Read the model definition and answer for the solid it produces. Units are mm, in the model's axes. Face numbers are marked on the shaded views. A direction names the side the tool comes from. Give positions to 0.01 mm unless a question says otherwise; leave off trailing zeros. Order: outer loops, then holes, each group sorted by start corner. A loop starts at its lowest first (then second) coordinate and runs counter-clockwise, first axis right, second up. Notation, with made-up numbers: (7, 56) -> (43, 56) arc R33 ccw to (43, 85) -> close; hole circle Ø2 at (65, 20.25). An arc over 180 degrees is marked (long way). Answer as CSV lines item,"result". Start each with the question number.
1) Find section A-A (x = 0). Determine the outline of the cut face in (y, z).
2) Find section D-D (y = -6.5). Determine the outline of the cut face in (x, z), and give its area (3 significant figures).
3) For the marked faces 4, 5 and 6, determine the directions among +Z, -Z, +X, -X, +Y, -Y from which every point of the face is accessible in a straight line to the end or side of a thin tool.
4) Find section C-C (x = -20.5). Determine the outline of the cut face in (y, z), and give its area (3 significant figures).
5) Straight lines are drawn through the part: L1, parallel to Z at x = -23, y = -10.35; L2, parallel to Z at x = -2, y = 18; L3, parallel to Z at x = 6, y = 2.5. For each, find the intervals that lie inside material, in ascending order. Write a range as from..to.
6) Flat-ended cylindrical pins translate along their axes: pin 1 Ø10 at (x, z) = (0.5, 41.5) entering from +Y; pin 2 Ø5 at (y, z) = (-10.5, 22) entering from -X; pin 3 Ø9.5 at (x, z) = (-18.5, 20.5) entering from +Y. Find the tip coordinate at first contact, or state that the pin passes through.
7) The mould has two halves that part along Y. Classify the marked faces 1, 2 and 3: +Y half, -Y half, draft (parallel to the pull), parting line (faces both ways), or undercut.
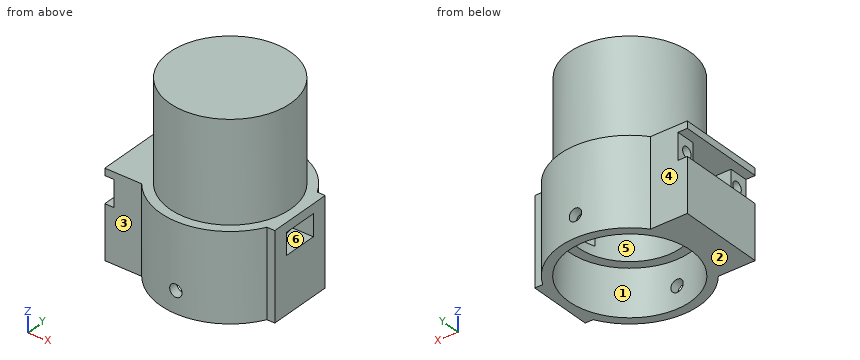
```python
from build123d import *

# Parameters (mm, degrees)
SKETCH_R        = 19.6
PAD_DEPTH       = 15
SKETCH001_R     = 16.5
PAD001_DEPTH    = 13
SKETCH002_W     = 11
SKETCH002_H     = 7
POCKET_DEPTH    = 10
SKETCH003_W     = 28
SKETCH003_H     = 8.5
POCKET001_DEPTH = 3
SKETCH004_R     = 1.75
SKETCH004_W     = 15.8
SKETCH004_H     = 8.5
POCKET002_DEPTH = 12
SKETCH006_R     = 2
HOLE_DEPTH      = 22.501
SKETCH007_R     = 2
HOLE001_DEPTH   = 22.501
SKETCH008_R     = 19.5
SKETCH008_R_2   = 16.5
PAD002_DEPTH    = 29
SKETCH009_R     = 19.5
PAD003_DEPTH    = 3


with BuildPart() as part:
    # Sketch → Pad (new body)
    with BuildSketch(Plane.XY):
        with BuildLine():
            Line((-29.5, 14), (-29.5, -14))
            Line((-29.5, -14), (-17.613915, -14))
            ThreePointArc((-17.613915, -14), (2.146366, -22.397391), (19.952193, -10.4))
            Line((19.952193, -10.4), (22.5, -10.4))
            Line((22.5, -10.4), (22.5, 10.4))
            Line((22.5, 10.4), (19.952193, 10.4))
            ThreePointArc((19.952193, 10.4), (2.146366, 22.397391), (-17.613915, 14))
            Line((-17.613915, 14), (-29.5, 14))
        make_face()
        Circle(SKETCH_R, mode=Mode.SUBTRACT)
    extrude(amount=PAD_DEPTH)

    # Sketch001 (on Face11 of Pad) → Pad001 (join)
    with BuildSketch(Plane.XY.offset(15)):
        with BuildLine():
            ThreePointArc((19.952193, 10.4), (2.146366, 22.397391), (-17.613915, 14))
            Line((-17.613915, 14), (-29.5, 14))
            Line((-29.5, 14), (-29.5, -14))
            Line((-29.5, -14), (-17.613915, -14))
            ThreePointArc((-17.613915, -14), (2.146366, -22.397391), (19.952193, -10.4))
            Line((22.5, -10.4), (19.952193, -10.4))
            Line((22.5, 10.4), (22.5, -10.4))
            Line((19.952193, 10.4), (22.5, 10.4))
        make_face()
        Circle(SKETCH001_R, mode=Mode.SUBTRACT)
    extrude(amount=PAD001_DEPTH)

    # Sketch002 (on Face10 of Pad001) → Pocket (cut)
    with BuildSketch(Plane.YZ.offset(22.5)):
        with Locations((0, 21.5)):
            Rectangle(SKETCH002_W, SKETCH002_H)
    extrude(amount=-POCKET_DEPTH, mode=Mode.SUBTRACT)

    # Sketch003 (on Face2 of Pocket) → Pocket001 (cut)
    with BuildSketch(Plane(origin=(-29.5, 0, 0), x_dir=(0, -1, 0), z_dir=(-1, 0, 0))):
        with Locations((0, 21.5)):
            Rectangle(SKETCH003_W, SKETCH003_H)
    extrude(amount=-POCKET001_DEPTH, mode=Mode.SUBTRACT)

    # Sketch004 (on Face12 of Pocket001) → Pocket002 (cut)
    with BuildSketch(Plane(origin=(-26.5, 0, 0), x_dir=(0, -1, 0), z_dir=(-1, 0, 0))):
        with Locations((10.35, 21.5)):
            Circle(SKETCH004_R)
        with Locations((-10.35, 21.5)):
            Circle(SKETCH004_R)
        with Locations((0, 21.5)):
            Rectangle(SKETCH004_W, SKETCH004_H)
    extrude(amount=-POCKET002_DEPTH, mode=Mode.SUBTRACT)

    # Sketch006 → Hole (cut, through all)
    with BuildSketch(Plane.XZ):
        with Locations((0, 7)):
            Circle(SKETCH006_R)
    extrude(amount=-HOLE_DEPTH, mode=Mode.SUBTRACT)

    # Sketch007 → Hole001 (cut, through all)
    with BuildSketch(Plane.XZ):
        with Locations((0, 7)):
            Circle(SKETCH007_R)
    extrude(amount=HOLE001_DEPTH, mode=Mode.SUBTRACT)

    # Sketch008 (on Face15 of Hole001) → Pad002 (join)
    with BuildSketch(Plane.XY.offset(28)):
        Circle(SKETCH008_R)
        Circle(SKETCH008_R_2, mode=Mode.SUBTRACT)
    extrude(amount=PAD002_DEPTH)

    # Sketch009 (on Face32 of Pad002) → Pad003 (join)
    with BuildSketch(Plane.XY.offset(57)):
        Circle(SKETCH009_R)
    extrude(amount=PAD003_DEPTH)


solid = part.part
```
Findings below:
1,outline,"(-22.5, 0) -> (-19.6, 0) -> (-19.6, 5) -> (-22.5, 5) -> close; (-22.5, 9) -> (-19.6, 9) -> (-19.6, 15) -> (-16.5, 15) -> (-16.5, 57) -> (16.5, 57) -> (16.5, 15) -> (19.6, 15) -> (19.6, 9) -> (22.5, 9) -> (22.5, 28) -> (19.5, 28) -> (19.5, 60) -> (-19.5, 60) -> (-19.5, 28) -> (-22.5, 28) -> close; (19.6, 0) -> (22.5, 0) -> (22.5, 5) -> (19.6, 5) -> close"
2,outline,"(-29.5, 0) -> (-18.49, 0) -> (-18.49, 15) -> (-15.17, 15) -> (-15.17, 17.25) -> (-29.5, 17.25) -> close; (-29.5, 25.75) -> (-15.17, 25.75) -> (-15.17, 57) -> (15.17, 57) -> (15.17, 15) -> (18.49, 15) -> (18.49, 0) -> (22.5, 0) -> (22.5, 28) -> (18.38, 28) -> (18.38, 60) -> (-18.38, 60) -> (-18.38, 28) -> (-29.5, 28) -> close"
2,area,"682 mm²"
3,face 4,"+Z, -Z, -X, +Y"
3,face 5,"-Z"
3,face 6,"+X, -X"
4,outline,"(-14, 0) -> (14, 0) -> (14, 28) -> (-14, 28) -> close; hole circle Ø3.5 at (-10.35, 21.5); hole (-7.9, 17.25) -> (7.9, 17.25) -> (7.9, 25.75) -> (-7.9, 25.75) -> close; hole circle Ø3.5 at (10.35, 21.5)"
4,area,"630 mm²"
5,L1,"0..19.75, 23.25..28"
5,L2,"15..60"
5,L3,"57..60"
6,pin 1,"y = 19.5"
6,pin 2,"x = -26.5"
6,pin 3,"y = 17.81"
7,face 1,"undercut"
7,face 2,"draft"
7,face 3,"-Y half"
